```python
from build123d import *

# Parameters (mm, degrees)
F0_W     = 22
F0_H     = 61
F1_DEPTH = 28
F3_DEPTH = 22.001
F5_DEPTH = 9


with BuildPart() as f1:
    # F0 (on Top) → F1 (new body)
    with BuildSketch(Plane.XY):
        with Locations((11, 30.5)):
            Rectangle(F0_W, F0_H)
    extrude(amount=F1_DEPTH)

    # F2 (on face) → F3 (cut, through all)
    with BuildSketch(Plane.YZ.offset(22)):
        Polygon((36, 28), (0, 28), (0, 10), align=None)
    extrude(amount=-F3_DEPTH, mode=Mode.SUBTRACT)

    # F4 (on face) → F5 (join)
    with BuildSketch(Plane(origin=(0, 0, 0), x_dir=(0, -1, 0), z_dir=(-1, 0, 0))):
        Polygon((-18, 19), (0, 10), (0, 19), align=None)
    extrude(amount=-F5_DEPTH)


solid = f1.part
```
Here's how the part is built. I have some questions about the finished solid (model axes, mm). A direction names the side the tool comes from. Coordinates: 2 decimals unless noted, no trailing zeros. Loops run counter-clockwise (first coordinate to the right, second up) from the corner with the lowest first, then second, coordinate; pieces in that order, holes last. Notation, with made-up numbers: (-17, 30.25) -> (-9, 30.25) arc R17 ccw to (-9, 37.25) -> close; hole circle Ø5 at (-13, -18). An arc over 180 degrees is marked (long way). Return JSON: item names as keys, results as strings.
1) If we section it at B-B, the plane y = 8.5: Write out the boundary of the cut face in (x, z).
Results below:
{"outline": "(0, 0) -> (22, 0) -> (22, 14.25) -> (9, 14.25) -> (9, 19) -> (0, 19) -> close"}
2) If we section it at D-D, the plane y = 31.5: Write out the boundary of the cut face in (x, z), then the cut area to 4 significant figures.
Results below:
{"outline": "(0, 0) -> (22, 0) -> (22, 25.75) -> (0, 25.75) -> close", "area": "566.5 mm²"}
3) If we section it at A-A, the plane z = 17.75: Write out the boundary of the cut face in (x, y).
Results below:
{"outline": "(0, 0) -> (9, 0) -> (9, 15.5) -> (22, 15.5) -> (22, 61) -> (0, 61) -> close"}
4) If we section it at C-C, the plane x = 9.75: Write out the boundary of the cut face in (y, z), then the cut area to 3 significant figures.
Results below:
{"outline": "(0, 0) -> (61, 0) -> (61, 28) -> (36, 28) -> (0, 10) -> close", "area": "1,380 mm²"}
5) For faces 1 (the face through (4, 9, 19)), 2 (the face through (8, 0, 7)), 3 (the face through (9, 5, 17)), which set-ups out of +Z, -Z, +X, -X, +Y, -Y let a thin tool reach every point of the face, with its end or its side?
Results below:
{"face 1": "+Z, +X, -X, -Y", "face 2": "+Z, -Z, +X, -X, -Y", "face 3": "+Z, +X, -Y"}
6) Will these pins go through, and if not, where does the flat tip stop? pin 1 (1.5 mm diameter, centred on x = 3, z = 21, fed in from -Y); pin 2 (2.5 mm diameter, centred on x = 5.5, y = 11.5, fed in from +Z).
Results below:
{"pin 1": "y = 20.5", "pin 2": "z = 19"}
7) I need wall thicknesses on line 1 (Z direction, x = 7.75, y = 15); line 2 (X direction, y = 11.5, z = 16.5); line 3 (Y direction, x = 14.5, z = 18.5). Which ranges of each line are inside material? Lowest first, please. Write a range as from..to.
Results below:
{"line 1": "0..19", "line 2": "0..9", "line 3": "17..61"}
